```python
from build123d import *
from build123d.topology import SkipClean

# Parameters (mm, degrees)
SKETCH1_R           = 1.5
BOSS_EXTRUDE1_DEPTH = 3
SKETCH2_OUTSIDE_W   = 28.48
SKETCH2_OUTSIDE_H   = 12.58
CUT_EXTRUDE1_DEPTH  = 12.743189516
BOSS_EXTRUDE2_START = -3
SKETCH3_R           = 1.5
BOSS_EXTRUDE2_DEPTH = 2


with BuildPart() as part:
    # Sketch1 → Boss-Extrude1 (new body)
    with BuildSketch(Plane(origin=(0, 0, 0), x_dir=(1, 0, 0), z_dir=(0, 1, 0))):
        with BuildLine():
            Line((-7.95, 3), (7.95, 3))
            ThreePointArc((7.95, 3), (10.95, 0), (7.95, -3))
            Line((7.95, -3), (-7.95, -3))
            ThreePointArc((-7.95, -3), (-10.95, 0), (-7.95, 3))
        make_face()
        with Locations(Location((-7.95, 0, 0), (0, 0, 270))):
            Circle(SKETCH1_R, mode=Mode.SUBTRACT)
        with Locations(Location((7.95, 0, 0), (0, 0, 270))):
            Circle(SKETCH1_R, mode=Mode.SUBTRACT)
    extrude(amount=BOSS_EXTRUDE1_DEPTH)

    # Sketch2 outside → Cut-Extrude1 (cut, through all)
    with SkipClean():  # the faces are left unmerged after this step: merging them gives an invalid solid
        with BuildSketch(Plane(origin=(0, 3, 0), x_dir=(1, 0, 0), z_dir=(0, 1, 0))):
            Rectangle(SKETCH2_OUTSIDE_W, SKETCH2_OUTSIDE_H)
            with BuildLine():
                ThreePointArc((-6.95625, 2.830629071), (-10.95, 0), (-6.95625, -2.830629071))
                ThreePointArc((-6.95625, -2.830629071), (0, -1.645032568), (6.95625, -2.830629071))
                ThreePointArc((6.95625, -2.830629071), (10.95, 0), (6.95625, 2.830629071))
                ThreePointArc((6.95625, 2.830629071), (0, 1.645032568), (-6.95625, 2.830629071))
            make_face(mode=Mode.SUBTRACT)
        extrude(amount=-CUT_EXTRUDE1_DEPTH, mode=Mode.SUBTRACT)

    # Sketch3 → Boss-Extrude2 (add)
    with SkipClean():  # the faces are left unmerged after this step: merging them gives an invalid solid
        with BuildSketch(Plane(origin=(0, 3, 0), x_dir=(1, 0, 0), z_dir=(0, 1, 0)).offset(BOSS_EXTRUDE2_START)):
            with BuildLine():
                ThreePointArc((-6.95625, -2.830629071), (-5.502424669, -1.734755026), (-4.95, 0))
                ThreePointArc((-4.95, 0), (-5.502424669, 1.734755026), (-6.95625, 2.830629071))
                ThreePointArc((-6.95625, 2.830629071), (-10.95, 0), (-6.95625, -2.830629071))
            make_face()
            with Locations(Location((-7.95, 0, 0), (0, 0, 270))):
                Circle(SKETCH3_R, mode=Mode.SUBTRACT)
            with BuildLine():
                ThreePointArc((6.95625, -2.830629071), (9.684755026, -2.447575331), (10.95, 0))
                ThreePointArc((10.95, 0), (9.684755026, 2.447575331), (6.95625, 2.830629071))
                ThreePointArc((6.95625, 2.830629071), (4.95, 0), (6.95625, -2.830629071))
            make_face()
            with Locations(Location((7.95, 0, 0), (0, 0, 270))):
                Circle(SKETCH3_R, mode=Mode.SUBTRACT)
        extrude(amount=-BOSS_EXTRUDE2_DEPTH)


solid = part.part
```
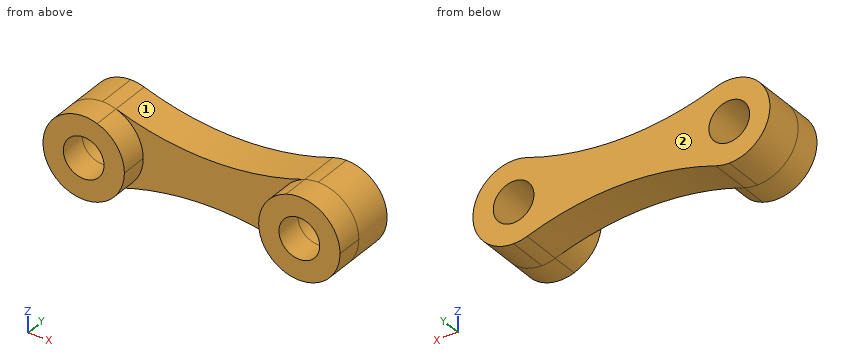
Check sheet for the modelled part. Datum: model origin and axes. Units: mm. Face numbers are marked on the shaded views. Coordinates: 2 decimals unless noted, no trailing zeros. Loops run counter-clockwise (first coordinate to the right, second up) from the corner with the lowest first, then second, coordinate; pieces in that order, holes last.
1) Material ranges on probe 1 along X at (y, z) = (2.3, 0); probe 2 along X at (y, z) = (-1.2, 0); probe 3 along X at (y, z) = (1.8, 1), recorded low to high.
2) Sectioned sample at A-A (y = -0.45). Record the boundary of the cut face in (x, z), and give its area (3 significant figures).
3) Sectioned sample at D-D (z = 2). Record the boundary of the cut face in (x, y), and give its area (3 significant figures).
4) Release check for a two-part mould opening along X. For the marked faces 1 and 2 record: released by +X, released by -X, zero draft, split by the parting line, or undercut.
5) Gauge pin test, flat ends, axial feed: pin 1 (2.5 mm diameter, centred on x = -7.95, z = 0, fed in from -Y); pin 2 (1.7 mm diameter, centred on x = 0.5, z = -0.5, fed in from -Y). Record the tip position at first contact, or that the pin passes through.
6) Sectioned sample at C-C (z = -0.5). Record the boundary of the cut face in (x, y).
7) Sectioned sample at B-B (y = 2). Record the boundary of the cut face in (x, z).
Check sheet entries:
1. probe 1: x = -10.95 to -9.45, -6.45 to 6.45, 9.45 to 10.95
1. probe 2: x = -10.95 to -9.45, -6.45 to -4.95, 4.95 to 6.45, 9.45 to 10.95
1. probe 3: x = -10.78 to -9.07, -6.83 to 6.83, 9.07 to 10.78
2. outline: circle Ø6 at (-7.95, 0); circle Ø6 at (7.95, 0); hole circle Ø3 at (-7.95, 0); hole circle Ø3 at (7.95, 0)
2. area: 42.4 mm2
3. outline: (-10.19, -2) - (-5.71, -2) - (-5.71, 0) - (-3.84, 0) - (-3.84, 3) - (-10.19, 3) - close; (3.84, 0) - (5.71, 0) - (5.71, -2) - (10.19, -2) - (10.19, 3) - (3.84, 3) - close
3. area: 55.9 mm2
4. face 1: undercut
4. face 2: zero draft
5. pin 1: passes through
5. pin 2: stops at y = 0
6. outline: (-10.91, -2) - (-9.36, -2) - (-9.36, 3) - (-10.91, 3) - close; (-6.54, -2) - (-4.99, -2) - (-4.99, 0) - (4.99, 0) - (4.99, -2) - (6.54, -2) - (6.54, 3) - (-6.54, 3) - close; (9.36, -2) - (10.91, -2) - (10.91, 3) - (9.36, 3) - close
7. outline: (-6.96, -2.83) arc R21 cw to (6.96, -2.83) arc R3 ccw (long way) to (6.96, 2.83) arc R21 cw to (-6.96, 2.83) arc R3 ccw (long way) to start; hole circle Ø3 at (-7.95, 0); hole circle Ø3 at (7.95, 0)
